Source: CAD feature listing. Evaluate the final solid. Frame: model axes, mm. A direction names the side the tool comes from. Coordinates: 2 decimals unless noted, no trailing zeros. Write each loop counter-clockwise with the first axis right and the second up, starting at its lowest first coordinate (ties: lowest second). Pieces come first, ordered by that corner, then holes. Notation, with made-up numbers: (57, 4) - (109, 4) arc R21 ccw to (109, 15) - close; hole circle Ø9 at (61.5, -21). An arc over 180 degrees is marked (long way). One line per question, with ' | ' between items.
Autodesk Inventor part; units mm, degrees
ref_plane "YZ Plane" through (0, 0, 0) normal (1, 0, 0) x (0, 1, 0)
ref_plane "XZ Plane" through (0, 0, 0) normal (0, 1, 0) x (-1, 0, 0)
ref_plane "XY Plane" through (0, 0, 0) normal (0, 0, 1) x (1, 0, 0)
sketch "スケッチ1" plane through (0, 0, 0) normal (1, 0, 0) x (0, 1, 0)
  line L0 (12, 0) -> (12, 5)
  line L1 (12, 5) -> (10, 5)
  line L2 (10, 5) -> (10, 22)
  line L3 (24, 20) -> (37.5, 20)
  line L4 (37.5, 20) -> (37.5, 0)
  line L5 (37.5, 0) -> (12, 0)
  line L6 (0, -4.4) -> (0, 26.4)
  line L7 (24, 20) -> (24, 22)
  line L8 (24, 22) -> (10, 22)
  point P0 (0, 0)
  dimension "d0" = 12
  dimension "d1" = 37.5
  dimension "d2" = 2
  dimension "d3" = 5
  dimension "d5" = 20
  dimension "d28" = 2
  dimension "d29" = 24
revolve "回転1" add sketch "スケッチ1" angle 360 about axis through (0, 0, -10) along (0, 0, 1)
chamfer "面取り1" distance 0.5 angle 45 1 edges at (0, -12, 0)
sketch "スケッチ2" plane through (0, 0, 20) normal (0, 0, 1) x (1, 0, 0)
  circle A0 centre (0, 0) radius 32
  point P0 (0, 32)
  point P1 (-27.7128, 16)
  point P2 (-27.7128, -16)
  point P3 (0, -32)
  point P4 (27.7128, -16)
  point P5 (27.7128, 16)
  dimension "d10" = 64
  dimension "d13" = 360
hole "穴1" at (0, 32, 20) at (-27.7128, 16, 20) at (-27.7128, -16, 20) at (0, -32, 20) at (27.7128, -16, 20) at (27.7128, 16, 20) direction (0, 0, -1) diameter 4.5 end through all
chamfer "面取り2" distance 1 angle 45 1 edges at (0, -37.5, 0)
chamfer "面取り3" distance 0.5 angle 45 1 edges at (0, -24, 22)
properties part number "unit-base2" material "ABS プラスチック"
Item 1: Ray query, line 1 along Y through (x, z) = (0, 9.75); line 2 along Y through (x, z) = (0, 1.75); line 3 along X through (y, z) = (0, 2.85). Return the intervals inside material, ascending. Write a range as [from, to].
Check sheet entries:
line 1: [-37.5, -34.25], [-29.75, -10], [10, 29.75], [34.25, 37.5] | line 2: [-37.5, -34.25], [-29.75, -12], [12, 29.75], [34.25, 37.5] | line 3: [-37.5, -12], [12, 37.5]
Item 2: Cut plane B-B on x = 0. State how many separate pieces and enclosed holes the cut face has, and give its area (4 significant figures).
Check sheet entries:
separate pieces: 4 | enclosed holes: 0 | area: 954.5 mm²
Item 3: Cut plane C-C on z = 4. Return loops of the section in (x, y), and give its area (3 significant figures).
Check sheet entries:
outline: circle Ø75 at (0, 0); hole circle Ø4.5 at (-27.71, -16); hole circle Ø4.5 at (-27.71, 16); hole circle Ø24 at (0, 0); hole circle Ø4.5 at (0, -32); hole circle Ø4.5 at (0, 32); hole circle Ø4.5 at (27.71, -16); hole circle Ø4.5 at (27.71, 16) | area: 3,870 mm²
Item 4: Mould query, pull axis Y, two halves, no side actions, for faces 4 (the face through (-1, 16, 0)), 5 (the face through (9.76, -2.17, 13.62)), 6 (the face through (-1.055, -23.977, 20.76)). Classes: pulls with the +Y half, pulls with the -Y half, needs draft (parallel to the pull), parting line crosses it, or undercut.
Check sheet entries:
face 4: needs draft | face 5: undercut | face 6: parting line crosses it
Item 5: Cut plane A-A on y = 0. Return loops of the section in (x, z), and give its area (3 significant figures).
Check sheet entries:
outline: (-37.5, 1) - (-36.5, 0) - (-12.5, 0) - (-12, 0.5) - (-12, 5) - (-10, 5) - (-10, 22) - (-23.5, 22) - (-24, 21.5) - (-24, 20) - (-37.5, 20) - close; (10, 5) - (12, 5) - (12, 0.5) - (12.5, 0) - (36.5, 0) - (37.5, 1) - (37.5, 20) - (24, 20) - (24, 21.5) - (23.5, 22) - (10, 22) - close | area: 1,130 mm²
Item 6: Access query for faces 1 (the face through (29.71, 14.96, 9.86)), 2 (the face through (-9, -5, 5)), 3 (the face through (24.5, -0.5, 20)). Directions: +Z, -Z, +X, -X, +Y, -Y. A direction counts if a zero-diameter tool reaches every point of the face in a straight line with its end or side. Return the directions, or none.
Check sheet entries:
face 1: +Z, -Z | face 2: -Z | face 3: +Z
Item 7: Pin query (flat end, axial travel): pin 1 Ø1 at (x, z) = (-24.5, 2.5) entering from +Y; pin 2 Ø3.5 at (x, y) = (-27.71, 16) entering from +Z; pin 3 Ø12 at (x, z) = (11, 12.5) entering from -Y; pin 4 Ø2 at (x, z) = (2, 7.5) entering from +Y. Return the tip coordinate at first contact, or that it passes through.
Check sheet entries:
pin 1: y = 28.81 | pin 2: through | pin 3: y = -37.17 | pin 4: y = 37.49
